```python
from build123d import *

# Parameters (mm, degrees)
SKETCH3_R           = 6.75
BOSS_EXTRUDE1_DEPTH = 12.5
SKETCH4_R           = 5
CUT_EXTRUDE1_DEPTH  = 10
SKETCH5_R           = 4.25
CUT_EXTRUDE2_DEPTH  = 43.343830719
RIB1_START          = -22
RIB1_DEPTH          = 15.341739823
RIB1_START_2        = 6.658260177
RIB1_2_DEPTH        = 15.341739823
RIB1_3_DEPTH        = 15.341739823
RIB1_4_DEPTH        = 15.341739823
SKETCH9_R           = 6.5
CUT_EXTRUDE3_DEPTH  = 44.637713047


with BuildPart() as part:
    # Sketch2 → Revolve1 (revolve)
    with BuildSketch(Plane(origin=(0, 0, 0), x_dir=(0, 0, -1), z_dir=(1, 0, 0)), mode=Mode.PRIVATE) as revolve1_sk:
        Polygon((0, 0), (26, 0), (26, 2.5), (23.8, 2.5), (23.8, 23.229829408), (26, 24.5), (26, 26), (21.4, 26), (21.4, 2.5), (0, 2.5), align=None)
    revolve(revolve1_sk.sketch.rotate(Axis((0, 2.5, 0), (0, -1, 0)), 180), axis=Axis((0, 2.5, 0), (0, -1, 0)))

    # Sketch3 → Boss-Extrude1 (add)
    with BuildSketch(Plane(origin=(0, 2.5, 0), x_dir=(1, 0, 0), z_dir=(0, 1, 0))):
        with Locations(Location((0, 0, 0), (0, 0, 90))):
            Circle(SKETCH3_R)
    extrude(amount=BOSS_EXTRUDE1_DEPTH)

    # Sketch4 → Cut-Extrude1 (cut)
    with BuildSketch(Plane(origin=(0, 15, 0), x_dir=(1, 0, 0), z_dir=(0, 1, 0))):
        with Locations(Location((0, 0, 0), (0, 0, 270))):
            Circle(SKETCH4_R)
    extrude(amount=-CUT_EXTRUDE1_DEPTH, mode=Mode.SUBTRACT)

    # Sketch5 → Cut-Extrude2 (cut, through all)
    with BuildSketch(Plane(origin=(0, 5, 0), x_dir=(1, 0, 0), z_dir=(0, 1, 0))):
        with Locations(Location((0, 0, 0), (0, 0, 270))):
            Circle(SKETCH5_R)
    extrude(amount=-CUT_EXTRUDE2_DEPTH, mode=Mode.SUBTRACT)

    # Rib1: read off the stored shape, not the designer's step
    # Rib1 outline → Rib1 (add)
    with BuildSketch(Plane.XY.offset(RIB1_START)):
        Polygon((1, 2.5), (1.109085847, 15), (-1.109085847, 15), (-1, 2.5), align=None)
    extrude(amount=RIB1_DEPTH)

    # Rib1 2 outline → Rib1 2 (add)
    with BuildSketch(Plane.XY.offset(RIB1_START_2)):
        Polygon((1, 2.5), (1.109085847, 15), (-1.109085847, 15), (-1, 2.5), align=None)
    extrude(amount=RIB1_2_DEPTH)

    # Rib1 3 outline → Rib1 3 (add)
    with BuildSketch(Plane.YZ.offset(RIB1_START)):
        Polygon((2.5, -1), (15, -1.109085847), (15, 1.109085847), (2.5, 1), align=None)
    extrude(amount=RIB1_3_DEPTH)

    # Rib1 4 outline → Rib1 4 (add)
    with BuildSketch(Plane.YZ.offset(RIB1_START_2)):
        Polygon((2.5, -1), (15, -1.109085847), (15, 1.109085847), (2.5, 1), align=None)
    extrude(amount=RIB1_4_DEPTH)

    # Sketch9 → Cut-Extrude3 (cut, through all)
    with BuildSketch(Plane(origin=(0, 2.5, 0), x_dir=(1, 0, 0), z_dir=(0, 1, 0))):
        with Locations(Location((-9.899494937, 9.899494937, 0), (0, 0, 270))):
            Circle(SKETCH9_R)
        with Locations(Location((9.899494937, -9.899494937, 0), (0, 0, 90))):
            Circle(SKETCH9_R)
        with Locations(Location((9.899494937, 9.899494937, 0), (0, 0, 270))):
            Circle(SKETCH9_R)
        with Locations(Location((-9.899494937, -9.899494937, 0), (0, 0, 90))):
            Circle(SKETCH9_R)
    extrude(amount=-CUT_EXTRUDE3_DEPTH, mode=Mode.SUBTRACT)


solid = part.part
```
Part model, mm, in its own coordinate system. A direction names the side the tool comes from. Give positions to 0.01 mm unless a question says otherwise; leave off trailing zeros. Order: outer loops, then holes, each group sorted by start corner. A loop starts at its lowest first (then second) coordinate and runs counter-clockwise, first axis right, second up. Notation, with made-up numbers: M 42,-24.75 L 96,-24.75 A29 cw 96,9.25 Z; hole C 5.5,34 d1. An arc over 180 degrees is marked long. Use a Markdown table: item, result. Add a question column.
(1) Saw through at C-C, the plane y = 14.25. Give the cut face in (x, z), and give its area (3 significant figures).
(2) Probe line 1 along X through (y, z) = (7.75, 0); line 2 along X through (y, z) = (5.5, -11.5); line 3 along Z through (x, y) = (10.5, 22.5). List the from-to ranges inside material, lowest first. Write a range as [from, to].
(3) Saw through at B-B, the plane z = 0. Give the cut face in (x, y).
(4) Saw through at D-D, the plane y = 20. Give the cut face in (x, z), and give its area (3 significant figures).
(5) 3-axis set-ups, long thin cutter, end or side, ignore diameter. For faces 4 (the face through (-16.085, 13.01, -17.542)), 5 (the face through (-7.95, 1.27, -3.7)): which of +Z, -Z, +X, -X, +Y, -Y reach the whole face in a straight line?
(6) Mould opens along Y. For faces 1 (the face through (7.95, 1.27, 3.7)), 2 (the face through (-4, 5, -2)), 3 (the face through (-7.19, 23.31, 22.83)) say: +Y half, -Y half, draft (parallel to the pull), parting line (faces both ways), or undercut.
(7) Drop flat-ended pins along their axis: P1, Ø8, axis at x = 2, z = -2.5, coming from the +Y side; P2, Ø1, axis at x = 8.5, y = 14.5, coming from the -Z side; P3, Ø6, axis at x = 5.5, y = 21.5, coming from the +Z side. Give the stop position or say it passes through.
(8) Saw through at A-A, the plane x = 0. Give the cut face in (y, z), and give its area (3 significant figures).
Answer key:
| question | item | result |
|---|---|---|
| 1 | outline | C 0,0 d47.6; hole M -21.37,-1.1 A21.4 ccw -1.1,-21.37 L -1.1,-6.66 A6.75 cw -6.66,-1.1 Z; hole M -21.37,1.1 L -6.66,1.1 A6.75 cw -1.1,6.66 L -1.1,21.37 A21.4 ccw Z; hole C 0,0 d10; hole M 1.1,-21.37 A21.4 ccw 21.37,-1.1 L 6.66,-1.1 A6.75 cw 1.1,-6.66 Z; hole M 1.1,6.66 A6.75 cw 6.66,1.1 L 21.37,1.1 A21.4 ccw 1.1,21.37 Z |
| 1 | area | 535 mm^2 |
| 2 | line 1 | [-23.8, -5], [5, 23.8] |
| 2 | line 2 | [-20.84, -18.05], [-1.03, 1.03], [18.05, 20.84] |
| 2 | line 3 | [-21.36, -18.65], [18.65, 21.36] |
| 3 | outline | M -26,0 L -4.25,0 L -4.25,5 L -5,5 L -5,15 L -21.4,15 L -21.4,26 L -26,26 L -26,24.5 L -23.8,23.23 L -23.8,2.5 L -26,2.5 Z; M 4.25,0 L 26,0 L 26,2.5 L 23.8,2.5 L 23.8,23.23 L 26,24.5 L 26,26 L 21.4,26 L 21.4,15 L 5,15 L 5,5 L 4.25,5 Z |
| 4 | outline | C 0,0 d47.6; hole C 0,0 d42.8 |
| 4 | area | 341 mm^2 |
| 5 | face 4 | none |
| 5 | face 5 | +Y, -Y |
| 6 | face 1 | draft |
| 6 | face 2 | +Y half |
| 6 | face 3 | undercut |
| 7 | P1 | y = 15 |
| 7 | P2 | z = -22.42 |
| 7 | P3 | z = 25.45 |
| 8 | outline | M 0,-26 L 2.5,-26 L 2.5,-23.8 L 23.23,-23.8 L 24.5,-26 L 26,-26 L 26,-21.4 L 15,-21.4 L 15,-5 L 5,-5 L 5,-4.25 L 0,-4.25 Z; M 0,4.25 L 5,4.25 L 5,5 L 15,5 L 15,21.4 L 26,21.4 L 26,26 L 24.5,26 L 23.23,23.8 L 2.5,23.8 L 2.5,26 L 0,26 Z |
| 8 | area | 645 mm^2 |
